Geometry check sheet. Reference: the model listing, model coordinates, mm. Coordinates: 2 decimals unless noted, no trailing zeros. Put each result on its own line as item: value.
Solid Edge part; units mm, degrees
sketch "Sketch1" plane through (0, 0, 0) normal (0, -1, 0) x (1, 0, 0)
  line L0 (-6, 8) -> (6, 8)
  line L1 (6, 8) -> (6, 0)
  line L2 (6, 0) -> (-6, 0)
  line L3 (-6, 0) -> (-6, 8)
  dimension "D1" = 6
  dimension "D2" = 6
extrude "Protrusion1" add sketch "Sketch1" along normal mid plane 390
sketch "Sketch2" plane through (0, 0, 8) normal (0, 0, 1) x (0, 1, 0)
  circle A0 centre (185, 0) radius 1.75
extrude "Cutout1" cut sketch "Sketch2" against normal through all
sketch "Sketch3" plane through (0, 0, 8) normal (0, 0, 1) x (0, 1, 0)
  circle A0 centre (185, 0) radius 3
extrude "ExtrudedCutout_2" cut sketch "Sketch3" against normal blind 4.5
pattern_linear "Pattern1" count 15 spacing 25 along (0, -1, 0) of "Cutout1", "ExtrudedCutout_2"
properties material "Stainless Steel, 410"
Q1. Section check A-A on z = 5.5. State how many separate pieces and enclosed holes the cut face has, then the cut area to 3 significant figures.
Answer block:
separate pieces: 1
enclosed holes: 15
area: 4,260 mm^2
Q2. Thickness scan on L1, parallel to X at y = 35, z = 6.9; L2, parallel to Z at x = 1, y = -37.5; L3, parallel to X at y = 85, z = 0.75. Record the ranges inside material, lowest first. Write a range as [from, to].
Answer block:
L1: x = [-6, -3], [3, 6]
L2: z = [0, 3.5]
L3: x = [-6, -1.75], [1.75, 6]
Q3. Depth check by flat-ended pin: pin 1 Ø5.5 at (x, y) = (0, -15) entering from +Z; pin 2 Ø7 at (x, y) = (0, -165) entering from -Z; pin 3 Ø1.8 at (x, y) = (0.5, 110) entering from +Z. Enter the tip coordinate at first touch or a pass-through.
Answer block:
pin 1: stops at z = 3.5
pin 2: stops at z = 0
pin 3: passes through
Q4. Draft check along Y on faces 1 (the flat face through (0, -195, 4)), 2 (the flat face through (2, 110, 3.5)), 3 (the flat face through (-6, 3, 4)), 4 (the flat face through (0, 8, 3.5)). Enter one of: pulls with the +Y half, pulls with the -Y half, needs draft (parallel to the pull), parting line crosses it, or undercut.
Answer block:
face 1: pulls with the -Y half
face 2: undercut
face 3: needs draft
face 4: undercut
